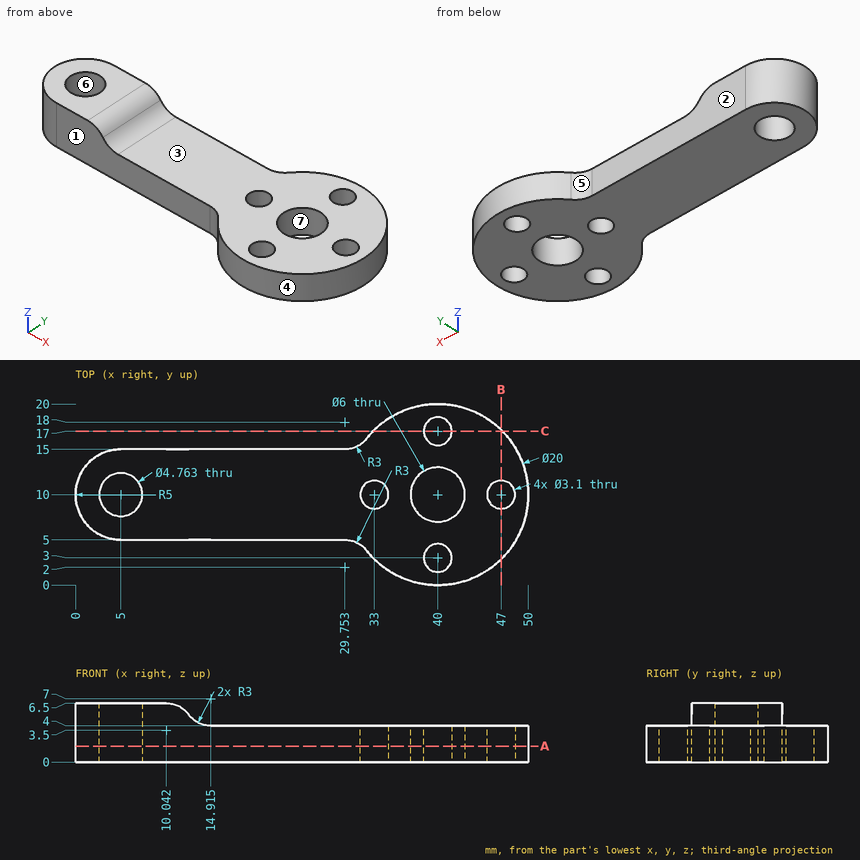
Study the drawing (mm; zero at the part's minimum x, y, z) and answer. A direction names the side the tool comes from. Round coordinates to 2 decimals unless told otherwise and drop trailing zeros. Write each loop counter-clockwise with the first axis right and the second up, starting at its lowest first coordinate (ties: lowest second). Pieces come first, ordered by that corner, then holes. Notation, with made-up numbers: (13.5, 36.5) - (21.5, 36.5) arc R26 ccw to (21.5, 64.5) - close; hole circle Ø2 at (79.25, -9). An arc over 180 degrees is marked (long way). Return JSON: item names as keys, results as strings. Group by question number.
Q1. The part is cut by section A-A on z = 1.75. Write down the section's boundary in (x, y), then the cut area to 3 significant figures.
Q2. For the marked faces 1, 2 and 3, determine the directions among +Z, -Z, +X, -X, +Y, -Y from which every point of the face is accessible in a straight line to the end or side of a thin tool.
Q3. The part is cut by section B-B on x = 47. Write down the section's boundary in (y, z).
Q4. Find the intervals of material crossed by L1, parallel to Y at x = 5, z = 3.25; L2, parallel to X at y = 8, z = 1.5 (1 decimal); L3, parallel to Z at x = 35, y = 7.25, in increasing order.
Q5. Each of these flat-tipped pins is pushed along its axis until it touches: pin 1 Ø4 at (x, y) = (38.5, 10) entering from +Z; pin 2 Ø3 at (y, z) = (15.5, 4) entering from -X; pin 3 Ø3 at (x, z) = (18, 3.5) entering from +Y. Where does it stop, or does it pass through?
Q6. The part is cut by section C-C on y = 17. Write down the section's boundary in (x, z).
Q7. The mould has two halves that part along Y. Classify the marked faces 4, 5, 6 and 7: released by +Y, released by -Y, zero draft, split by the parting line, or undercut.
Solved:
{
 "1": {"outline": "(5, 5) - (29.75, 5) arc R3 cw to (32.12, 3.85) arc R10 ccw (long way) to (32.12, 16.15) arc R3 cw to (29.75, 15) - (5, 15) arc R5 ccw to start; hole circle Ø4.76 at (5, 10); hole circle Ø3.1 at (33, 10); hole circle Ø6 at (40, 10); hole circle Ø3.1 at (40, 3); hole circle Ø3.1 at (40, 17); hole circle Ø3.1 at (47, 10)", "area": "532 mm²"},
 "2": {"face 1": "+Z, -Z, -X, -Y", "face 2": "+Z, -Z, -X, +Y", "face 3": "+Z, +X, +Y, -Y"},
 "3": {"outline": "(2.86, 0) - (8.45, 0) - (8.45, 4) - (2.86, 4) - close; (11.55, 0) - (17.14, 0) - (17.14, 4) - (11.55, 4) - close"},
 "4": {"L1": "5 to 7.62, 12.38 to 15", "L2": "0.4 to 3.7, 6.3 to 37.8, 42.2 to 49.8", "L3": "0 to 4"},
 "5": {"pin 1": "z = 4", "pin 2": "x = 2", "pin 3": "y = 15"},
 "6": {"outline": "(32.86, 0) - (38.45, 0) - (38.45, 4) - (32.86, 4) - close; (41.55, 0) - (47.14, 0) - (47.14, 4) - (41.55, 4) - close"},
 "7": {"face 4": "split by the parting line", "face 5": "released by +Y", "face 6": "undercut", "face 7": "undercut"}
}
